Build history of the part. All positions in model axes, mm. Face numbers are marked on the shaded views. A direction names the side the tool comes from. Round coordinates to 2 decimals unless told otherwise and drop trailing zeros. Loops run counter-clockwise (first coordinate to the right, second up) from the corner with the lowest first, then second, coordinate; pieces in that order, holes last. Notation, with made-up numbers: (76.25, -31.75) - (110.25, -31.75) arc R21 ccw to (110.25, -10.75) - close; hole circle Ø10 at (67, 28.5). An arc over 180 degrees is marked (long way). Use one line per item in the form item = value. Start each with the question number.
Q1. Saw through at B-B (z = -3). Give the cut face in (x, y), then the cut area to 3 significant figures.
Q2. Saw through at C-C (y = 5). Give the cut face in (x, z).
Q3. Mould opens along X. For the marked faces 1, 2 and 3 say: released by +X, released by -X, zero draft, split by the parting line, or undercut.
Q4. Saw through at A-A (x = -3). Give the cut face in (y, z), then the cut area to 3 significant figures.
Q5. 3-axis set-ups, long thin cutter, end or side, ignore diameter. For the marked faces 4, 5 and 6: which of +Z, -Z, +X, -X, +Y, -Y reach the whole face in a straight line?
Q6. Saw through at D-D (z = 13). Give the cut face in (x, y) (3 decimals), then the cut area to 3 significant figures.
Q7. Drill centre lines: line 1 (Z direction, x = -4.25, y = -2.25); line 2 (Y direction, x = 0, z = -13.05) (3 decimals); line 3 (Y direction, x = 0, z = -11.55) (3 decimals). Where is each one in solid material? Low to high.
Q8. Pin check, flat tips, straight feed: pin 1 (4.5 mm diameter, centred on x = 1, y = 6.5, fed in from +Z); pin 2 (1.4 mm diameter, centred on x = -5.5, z = 1.5, fed in from +Y); pin 3 (5 mm diameter, centred on y = 5.5, z = 14, fed in from +X). Stop position of each tip, or through.
```python
from build123d import *

# Parameters (mm, degrees)
SKETCH1_W                      = 14
SKETCH1_H                      = 15
BOSS_EXTRUDE1_DEPTH            = 5
SKETCH3_R                      = 1.1
CUT_EXTRUDE1_DEPTH             = 14
BOSS_EXTRUDE2_DEPTH            = 4.3
SKETCH5_R                      = 1.125
CUT_EXTRUDE2_DEPTH             = 4.3
FILLET1_R                      = 2.5
CUT_EXTRUDE3_REACH             = 22.227
CUT_EXTRUDE3_DIRECTION_2_REACH = 22.227
BOSS_EXTRUDE4_START            = -14
SKETCH7_R                      = 1.1
BOSS_EXTRUDE4_DEPTH            = 3.6
BOSS_EXTRUDE5_START            = -10.4
SKETCH8_R                      = 1.1
BOSS_EXTRUDE5_DEPTH            = 10.4
FILLET2_R                      = 10


with BuildPart() as part:
    # Sketch1 → Boss-Extrude1 (new body)
    with BuildSketch(Plane(origin=(0, 0, 0), x_dir=(1, 0, 0), z_dir=(0, 1, 0))):
        with Locations((0, 7.5)):
            Rectangle(SKETCH1_W, SKETCH1_H)
    extrude(amount=-BOSS_EXTRUDE1_DEPTH)

    # Sketch3 → Cut-Extrude1 (cut)
    with BuildSketch(Plane.ZY.offset(7)):
        with Locations((-12.5, -2.5)):
            Circle(SKETCH3_R)
    extrude(amount=-CUT_EXTRUDE1_DEPTH, mode=Mode.SUBTRACT)

    # Sketch4 → Boss-Extrude2 (add)
    with BuildSketch(Plane(origin=(0, 0, -15), x_dir=(-1, 0, 0), z_dir=(0, 0, -1))):
        with BuildLine():
            Line((-7, 0), (-3.763056055, 8.981248181))
            ThreePointArc((-3.763056055, 8.981248181), (0, 11.625), (3.763056055, 8.981248181))
            Line((3.763056055, 8.981248181), (7, 0))
            Line((7, 0), (-7, 0))
        make_face()
    extrude(amount=-BOSS_EXTRUDE2_DEPTH)

    # Sketch5 → Cut-Extrude2 (cut)
    with BuildSketch(Plane(origin=(0, 0, -15), x_dir=(-1, 0, 0), z_dir=(0, 0, -1))):
        with Locations((0, 7.625)):
            Circle(SKETCH5_R)
    extrude(amount=-CUT_EXTRUDE2_DEPTH, mode=Mode.SUBTRACT)

    # Fillet1
    fillet1_edges = [part.edges().sort_by_distance(p)[0] for p in [
        (0, -5, -15),
        (0, 0, -10.7),
    ]]
    fillet(fillet1_edges, radius=FILLET1_R)

    # Sketch6 → Cut-Extrude3 (cut, up to next)
    with BuildSketch(Plane(origin=(0, 0, 0), x_dir=(1, 0, 0), z_dir=(0, 1, 0)), mode=Mode.PRIVATE) as cut_extrude3_sk1:
        with BuildLine():
            Line((-3.5, -5.5), (-3.5, 5.5))
            ThreePointArc((-3.5, 5.5), (0, 9), (3.5, 5.5))
            Line((3.5, 5.5), (3.5, -5.5))
            ThreePointArc((3.5, -5.5), (0, -9), (-3.5, -5.5))
        make_face()
    cut_extrude3_tool1 = extrude(cut_extrude3_sk1.sketch, amount=-CUT_EXTRUDE3_REACH, mode=Mode.PRIVATE) & part.part
    add(cut_extrude3_tool1.solids().sort_by_distance((0, 0, 0))[0], mode=Mode.SUBTRACT)

    # Sketch6 → Cut-Extrude3 direction 2 (cut, up to next)
    with BuildSketch(Plane(origin=(0, 0, 0), x_dir=(1, 0, 0), z_dir=(0, 1, 0)), mode=Mode.PRIVATE) as cut_extrude3_direction_2_sk1:
        with BuildLine():
            Line((-3.5, -5.5), (-3.5, 5.5))
            ThreePointArc((-3.5, 5.5), (0, 9), (3.5, 5.5))
            Line((3.5, 5.5), (3.5, -5.5))
            ThreePointArc((3.5, -5.5), (0, -9), (-3.5, -5.5))
        make_face()
    cut_extrude3_direction_2_tool1 = extrude(cut_extrude3_direction_2_sk1.sketch, amount=CUT_EXTRUDE3_DIRECTION_2_REACH, mode=Mode.PRIVATE) & part.part
    add(cut_extrude3_direction_2_tool1.solids().sort_by_distance((0, 0, 0))[0], mode=Mode.SUBTRACT)

    # Mirror1: part across plane


with BuildPart() as part_1:
    add(part.part)
    add(part.part.mirror(Plane.XY))

    # Sketch7 → Boss-Extrude4 (add)
    with BuildSketch(Plane(origin=(7, 0, 0), x_dir=(0, 0, -1), z_dir=(1, 0, 0)).offset(BOSS_EXTRUDE4_START)):
        with BuildLine():
            Line((-12.5, -5), (-18.5, -5))
            ThreePointArc((-18.5, -5), (-21, -2.5), (-18.5, 0))
            Line((-18.5, 0), (-12.5, 0))
            ThreePointArc((-12.5, 0), (-10, -2.5), (-12.5, -5))
        make_face()
        with Locations((-18, -2.5)):
            Circle(SKETCH7_R, mode=Mode.SUBTRACT)
    extrude(amount=BOSS_EXTRUDE4_DEPTH)

    # Sketch8 → Boss-Extrude5 (add)
    with BuildSketch(Plane(origin=(7, 0, 0), x_dir=(0, 0, -1), z_dir=(1, 0, 0)).offset(BOSS_EXTRUDE5_START)):
        with Locations((-12.5, -2.5)):
            Circle(SKETCH8_R)
    extrude(amount=BOSS_EXTRUDE5_DEPTH)

    # Fillet2
    # the kernel refuses this fillet: 10 mm, written as the material it adds along each edge
    with BuildSketch(Plane(origin=(-7, 0, 15), x_dir=(0, 1, 0), z_dir=(1, 0, 0))) as fillet2_piece_1_section:
        with BuildLine():
            CenterArc((8.177078252, 10), FILLET2_R, 211.332251498, 58.667748502)
            Line((-0.36458435, 4.8), (-1.21875061, 4.28))
            ThreePointArc((-1.21875061, 4.28), (-1, 3.5), (-1, 0))
            Line((-1, 0), (0, -1))
            Line((0, -1), (8.177078252, -1))
            Line((8.177078252, -1), (8.177078252, 0))
        make_face()
    fillet2_piece_1 = extrude(amount=3.6, mode=Mode.PRIVATE)
    fillet2_piece_1 = split(fillet2_piece_1, bisect_by=Plane(origin=(-6.281736491, 1.992899149, 16.030712871), z_dir=(0.9407640136683284, -0.33906204533485823, 0)), keep=Keep.TOP, mode=Mode.PRIVATE)
    add(fillet2_piece_1)


solid = part_1.part
```
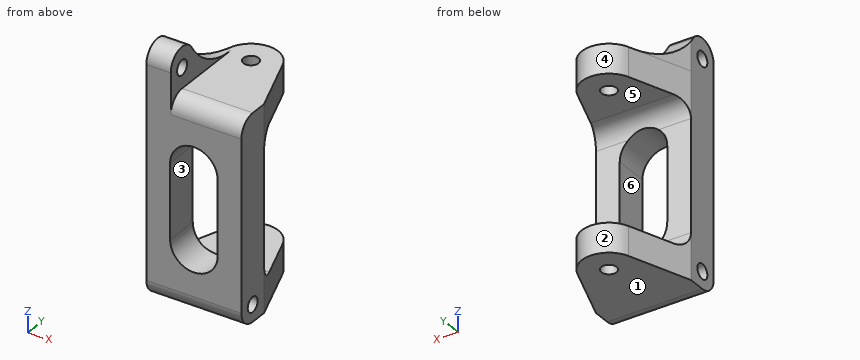
Report:
q1.outline = (-7, -5) - (-3.5, -5) - (-3.5, 0) - (-7, 0) - close; (3.5, -5) - (7, -5) - (7, 0) - (3.5, 0) - close
q1.area = 35.0 mm²
q2.outline = (-5.2, -15) - (5.2, -15) - (5.2, -10.7) - (-5.2, -10.7) - close; (-5.2, 10.7) - (5.2, 10.7) - (5.2, 15) - (-3.4, 15) - (-3.4, 15.52) - (-5.2, 15.52) - close
q3.face_1 = zero draft
q3.face_2 = split by the parting line
q3.face_3 = undercut
q4.outline = (-5, -12.5) arc R2.5 ccw to (-2.5, -15) - (10.27, -15) - (10.27, -10.7) - (2.5, -10.7) arc R2.5 cw to (0, -8.2) - (0, -7.3) - (-5, -7.3) - close; (-5, 7.3) - (0, 7.3) - (0, 8.2) arc R2.5 cw to (2.5, 10.7) - (10.27, 10.7) - (10.27, 15) - (-2.5, 15) arc R2.5 ccw to (-5, 12.5) - close; hole circle Ø2.2 at (-2.5, -12.5)
q4.area = 161 mm²
q5.face_4 = +Z, -Z, +Y
q5.face_5 = +X, -X, +Y
q5.face_6 = +Y, -Y
q6.outline = (-7, -5) - (-3.4, -5) - (-3.4, -4.949) - (7, -4.949) - (7, 0) - (3.763, 8.981) arc R4 ccw to (-3.763, 8.981) - (-7, 0) - close; hole circle Ø2.25 at (0, 7.625)
q6.area = 177 mm²
q7.line_1 = -15 to -13.57, -11.43 to 16.93, 19.07 to 20.99
q7.line_2 = -4.939 to -3.453, -1.547 to 6.5, 8.75 to 11.625
q7.line_3 = -5 to -3.055, -1.945 to 6.5, 8.75 to 11.625
q8.pin_1 = 15
q8.pin_2 = 0
q8.pin_3 = 5.92
